Geometry: final body of the model. Coordinates: model frame, mm. A direction names the side the tool comes from. Coordinates: 2 decimals unless noted, no trailing zeros. Loops run counter-clockwise (first coordinate to the right, second up) from the corner with the lowest first, then second, coordinate; pieces in that order, holes last. Notation, with made-up numbers: (-30.5, -16) - (2.5, -16) arc R17 ccw to (2.5, -7) - close; hole circle Ø4 at (-14.5, -12.5). An arc over 180 degrees is marked (long way). Put each result on its own line as item: value. Start each with the question number.
1) Section A-A on x = 54. Output: boundary loops of the cut face in (y, z).
2) Draft query along Y for faces 5 (the flat face through (41, -3, 10)), 6 (the flat face through (50.662, -40.957, 7.535)), 7 (the flat face through (41.87, -46.31, 7.53)). Return one class per face: +Y half, -Y half, draft (parallel to the pull), parting line (faces both ways), or undercut.
3) Material intervals for line 1 along Y through (x, z) = (43, 9.5); line 2 along Y through (x, z) = (31, 9.25); line 3 along Y through (x, z) = (35.5, 9.7), sorted ascending. Write a range as from..to.
4) Section D-D on y = 59.5. Output: boundary loops of the cut face in (x, z), and give its area (3 significant figures).
5) Section C-C on x = 41. Output: boundary loops of the cut face in (y, z).
6) Section B-B on z = 6. Output: boundary loops of the cut face in (x, y).
7) Reachability of faces 1 (the flat face through (35.23, 38.65, 7.53)), 2 (the flat face through (25, 42.674, 8)), 3 (the flat face through (46.4, 3.6, 7.5)), 4 (the flat face through (27.174, 66, 8)) from +Z, -Z, +X, -X, +Y, -Y: full face, straight path, thin tool, end or side. Return the list, or none.
8) Contact query for flat-ended pins moving along their axis: pin 1 Ø1.5 at (x, z) = (24, 6.5) entering from -Y; pin 2 Ø0.9 at (y, z) = (65.5, 7) entering from +X; pin 3 Ø0.8 at (y, z) = (43.5, 8) entering from +X; pin 4 Ø4 at (x, y) = (29.84, -25.3) entering from -Z. Output: stop coordinate, or through.
```python
from build123d import *

# Parameters (mm, degrees)
F0_R     = 1.7
F1_DEPTH = 5
F2_ANGLE = 180


with BuildPart() as f1:
    # F0 (on Top) → F1 (new body)
    with BuildSketch(Plane.XY):
        with BuildLine():
            Line((14.554017, 67.673713), (9.554017, 67.673713))
            Line((9.554017, 67.673713), (9.554017, 64.673713))
            Line((9.554017, 64.673713), (-19.124805, 23.716111))
            Line((-19.124805, 23.716111), (0.01047, -17.012764))
            Line((0.01047, -17.012764), (0.01047, -27.012764))
            Line((0.01047, -27.012764), (7.081537, -34.083832))
            Line((7.081537, -34.083832), (11.377259, -29.78811))
            ThreePointArc((11.377259, -29.78811), (13.142242, -26.391636), (12.634428, -22.597782))
            Line((12.634428, -22.597782), (-9.124805, 23.716111))
            Line((-9.124805, 23.716111), (-3.120972, 32.290473))
            Line((-3.120972, 32.290473), (6.244902, 45.185738))
            ThreePointArc((6.244902, 45.185738), (8.385212, 45.49281), (9.554017, 43.673713))
            Line((9.554017, 43.673713), (9.554017, 42.673713))
            Line((9.554017, 42.673713), (14.554017, 42.673713))
            Line((14.554017, 42.673713), (14.554017, 67.673713))
        make_face()
        with Locations((6.887131, -25.297982)):
            Circle(F0_R, mode=Mode.SUBTRACT)
        with BuildLine():
            Line((7.081537, -34.083832), (0.01047, -27.012764))
            Line((0.01047, -27.012764), (-28.273802, -55.297035))
            Line((-28.273802, -55.297035), (-25.940349, -57.630488))
            ThreePointArc((-25.940349, -57.630488), (-24.087706, -57.261974), (-23.038268, -58.832569))
            ThreePointArc((-23.038268, -58.832569), (-23.167673, -59.483131), (-23.536186, -60.034651))
            Line((-23.536186, -60.034651), (-21.202734, -62.368103))
            Line((-21.202734, -62.368103), (7.081537, -34.083832))
        make_face()
        with BuildLine():
            Line((-25.940349, -57.630488), (-28.273802, -55.297035))
            ThreePointArc((-28.273802, -55.297035), (-28.273802, -62.368103), (-21.202734, -62.368103))
            Line((-21.202734, -62.368103), (-23.536186, -60.034651))
            ThreePointArc((-23.536186, -60.034651), (-25.940349, -60.034651), (-25.940349, -57.630488))
        make_face()
    extrude(amount=F1_DEPTH)


with BuildPart() as f1_1:
    # F2: moved
    add(f1.part.rotate(Axis((14.554017, 55.173713, 5), (0, -1, 0)), F2_ANGLE))


with BuildPart() as f1_2:
    # F3: moved
    add(f1_1.part.moved(Location((7.62, 0, 0))))


solid = f1_2.part
```
Answer block:
1. outline: (-58.44, 5) - (-44.3, 5) - (-44.3, 10) - (-58.44, 10) - close; (19.77, 5) - (26.36, 5) - (26.36, 10) - (19.77, 10) - close
2. face 5: draft
2. face 6: undercut
2. face 7: -Y half
3. line 1: y = -47.44..-33.3, -3.64..17.64, 27.79..42.07
3. line 2: y = -35.44..-26.54, -24.05..-7.9, 44.47..59.21
3. line 3: y = -39.94..1.68, 38.28..52.78
4. outline: (22.17, 5) - (30.8, 5) - (30.8, 10) - (22.17, 10) - close
4. area: 43.1 mm²
5. outline: (-45.44, 5) - (-31.3, 5) - (-31.3, 10) - (-45.44, 10) - close; (-7.9, 5) - (13.39, 5) - (13.39, 10) - (-7.9, 10) - close; (30.65, 5) - (44.93, 5) - (44.93, 10) - (30.65, 10) - close
6. outline: (22.17, 42.67) - (27.17, 42.67) - (27.17, 43.67) arc R2 cw to (30.48, 45.19) - (39.85, 32.29) - (45.85, 23.72) - (24.09, -22.6) arc R6.35 ccw to (25.35, -29.79) - (57.93, -62.37) arc R5 ccw to (65, -55.3) - (36.72, -27.01) - (36.72, -17.01) - (55.85, 23.72) - (27.17, 64.67) - (27.17, 67.67) - (22.17, 67.67) - close; hole circle Ø3.4 at (29.84, -25.3); hole (59.77, -58.83) arc R1.7 ccw to (60.26, -60.03) arc R1.7 ccw (long way) to start
7. face 1: +Z, -Z
7. face 2: +Z, -Z, -X
7. face 3: +Z, -Z, +X
7. face 4: +Z, -Z, +X, +Y
8. pin 1: stops at y = -29.09
8. pin 2: stops at x = 27.17
8. pin 3: stops at x = 42.28
8. pin 4: stops at z = 5
